Design review of the part shown in the three views and the two pictorial views. Dimensions are in mm from the part's minimum x, y and z. A direction names the side the tool comes from. Give positions to 0.01 mm unless a question says otherwise; leave off trailing zeros. Loops run counter-clockwise (first coordinate to the right, second up) from the corner with the lowest first, then second, coordinate; pieces in that order, holes last. Notation, with made-up numbers: (24, 56) - (58, 56) arc R19 cw to (58, 89) - close; hole circle Ø5 at (74, 81). An arc over 180 degrees is marked (long way). Answer as a JSON object with one key per item and string values.
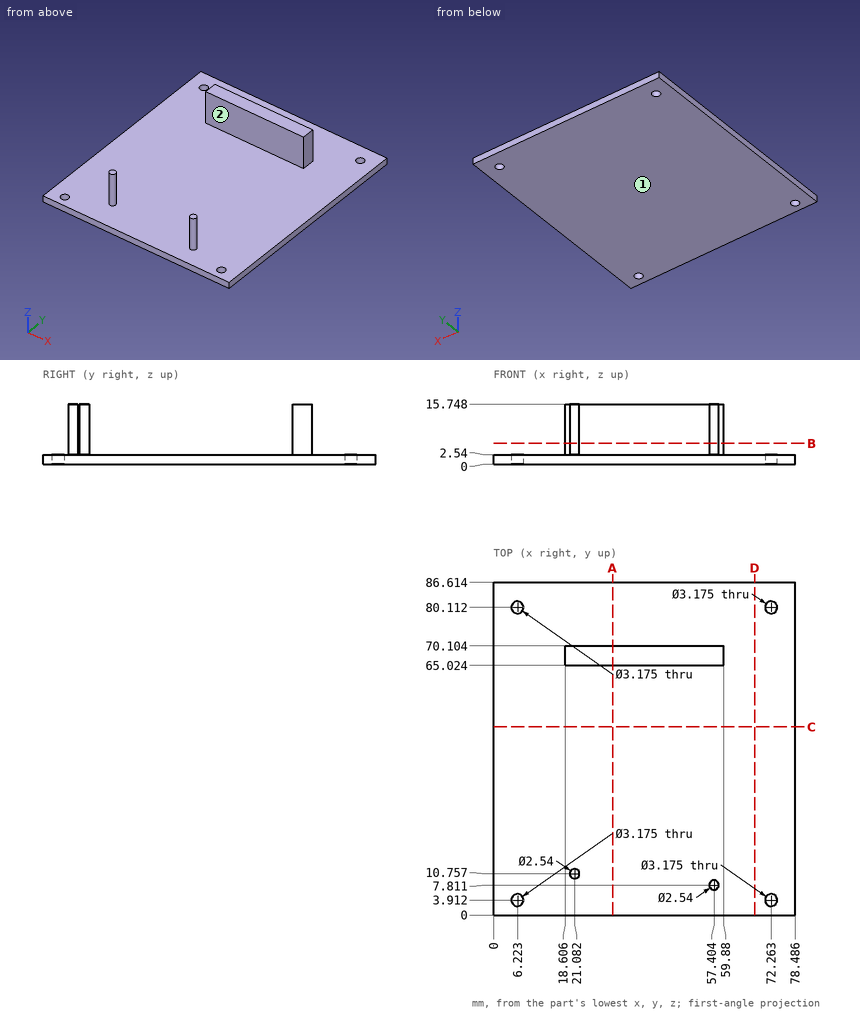
Q1. For the marked faces 1 and 2, list the 3-axis set-ups (+Z, -Z, +X, -X, +Y, -Y) from which the entire face can be reached by the end or side of a thin tool; tool diameter is ignored.
Results:
{"face 1": "-Z, +X, -X, +Y, -Y", "face 2": "+Z, +X, -X"}
Q2. Consider section B-B, the plane z = 5.5. State the section outline as (x, y) points (1 decimal).
Results:
{"outline": "(18.6, 65) - (59.9, 65) - (59.9, 70.1) - (18.6, 70.1) - close; circle Ø2.5 at (21.1, 10.8); circle Ø2.5 at (57.4, 7.8)"}
Q3. Clearance check with flat-ended pins moving along their axes: pin 1 Ø4 at (x, y) = (6.22, 80.11) entering from +Z; pin 2 Ø5.5 at (y, z) = (67.5, 9) entering from +X; pin 3 Ø6.5 at (x, z) = (45, 12) entering from -Y. State where each tip first meets the part, or that it passes through.
Results:
{"pin 1": "stops at z = 2.54", "pin 2": "stops at x = 59.88", "pin 3": "stops at y = 65.02"}
Q4. Consider section A-A, the plane x = 31. State the section outline as (y, z) points (1 decimal), plus the area to 3 significant figures.
Results:
{"outline": "(0, 0) - (86.6, 0) - (86.6, 2.5) - (70.1, 2.5) - (70.1, 15.7) - (65, 15.7) - (65, 2.5) - (0, 2.5) - close", "area": "287 mm^2"}
Q5. To check wall thickness, follow probe 1 along Y at (x, z) = (38.5, 5.75) (1 decimal); probe 2 along Y at (x, z) = (20, 11.5) (1 decimal); probe 3 along Z at (x, y) = (14, 45). State the ranges of each line that lie inside material, in increasing order. Write a range as [from, to].
Results:
{"probe 1": "y = [65, 70.1]", "probe 2": "y = [10.1, 11.4], [65, 70.1]", "probe 3": "z = [0, 2.54]"}
Q6. Consider section C-C, the plane y = 49. State the section outline as (x, z) points (1 decimal).
Results:
{"outline": "(0, 0) - (78.5, 0) - (78.5, 2.5) - (0, 2.5) - close"}
Q7. Consider section D-D, the plane x = 68. State the section outline as (y, z) points (1 decimal).
Results:
{"outline": "(0, 0) - (86.6, 0) - (86.6, 2.5) - (0, 2.5) - close"}
